Could you check a few things on this model? Use its own coordinates, in mm. Face numbers are marked on the shaded views. A direction names the side the tool comes from. Round coordinates to 2 decimals unless told otherwise and drop trailing zeros. Loops run counter-clockwise (first coordinate to the right, second up) from the corner with the lowest first, then second, coordinate; pieces in that order, holes last. Notation, with made-up numbers: M -37,8.25 L -28,8.25 A32 ccw -28,37.25 Z; hole C 70,32 d3. An arc over 180 degrees is marked long. One line per item, written item: value. Start each with the question number.
Q1. Imagine slicing it at B-B (x = 13). Please give me the cut outline in (y, z).
Q2. Thinking about a two-plate mould opening in Z: for the marked faces 1, 2 and 3, which applies, released by +Z, released by -Z, zero draft, split by the parting line, or undercut?
Q3. Please list where these lines run through material, in increasing order: line 1 along Z through (x, y) = (10.75, 40); line 2 along Z through (x, y) = (1, 4); line 3 along Y through (x, z) = (16, 1.65).
Q4. Imagine slicing it at A-A (z = 7). Please give me the cut outline in (x, y), then the cut area to 3 significant figures.
Q5. Imagine slicing it at D-D (z = 17.25). Please give me the cut outline in (x, y).
Q6. Imagine slicing it at C-C (y = 19). Please give me the cut outline in (x, z), then the cut area to 3 significant figures.
Q7. I'm going to push flat-ended pins straight in: pin 1 Ø2 at (y, z) = (40, 22) entering from -X; pin 2 Ø1.5 at (x, y) = (25.5, 25) entering from +Z; pin 3 Ø3 at (y, z) = (5, 21) entering from +X; pin 4 Ø1.5 at (x, z) = (24, 19) entering from -Y. Where does each tip first touch, or does it pass through?
Q8. Which directions (+Z, -Z, +X, -X, +Y, -Y) give clear straight access to the entire face, cutting with the end or side of a thin tool? Please do the marked faces 4, 5 and 6.
from build123d import *

# Parameters (mm, degrees)
SKETCH002_R     = 3.1
PAD001_DEPTH    = 20
PAD_DEPTH       = 30
SKETCH001_R     = 13
POCKET_DEPTH    = 27
SKETCH003_R     = 1.7
POCKET001_DEPTH = 3
SKETCH004_R     = 3.6
SKETCH004_R_2   = 1.7
POCKET002_DEPTH = 3


with BuildPart() as pad001:
    # Sketch002 → Pad001 (new body)
    with BuildSketch(Plane.YZ.offset(3)):
        with Locations((4, 22)):
            Circle(SKETCH002_R)
        with Locations((40, 22)):
            Circle(SKETCH002_R)
        with Locations((4, 8)):
            Circle(SKETCH002_R)
        with Locations((40, 8)):
            Circle(SKETCH002_R)
    extrude(amount=PAD001_DEPTH)


with BuildPart() as pocket002:
    # Sketch → Pad (new body)
    with BuildSketch(Plane.XY):
        with BuildLine():
            Line((0, 0), (0, 44))
            Line((0, 44), (3, 44))
            Line((3, 44), (21.975605, 35.758343))
            ThreePointArc((21.975609, 8.241648), (31, 21.999997), (21.975605, 35.758343))
            Line((21.975609, 8.241648), (3, 0))
            Line((3, 0), (0, 0))
        make_face()
    extrude(amount=PAD_DEPTH)

    # Sketch001 → Pocket (cut)
    with BuildSketch(Plane.XY.offset(30)):
        with Locations((16, 22)):
            Circle(SKETCH001_R)
    extrude(amount=-POCKET_DEPTH, mode=Mode.SUBTRACT)

    # Cut: cut Pad001
    add(pad001.part, mode=Mode.SUBTRACT)

    # Sketch003 → Pocket001 (cut)
    with BuildSketch(Plane.YZ.offset(3)):
        with Locations((4, 22)):
            Circle(SKETCH003_R)
        with Locations((40, 22)):
            Circle(SKETCH003_R)
        with Locations((4, 8)):
            Circle(SKETCH003_R)
        with Locations((40, 8)):
            Circle(SKETCH003_R)
    extrude(amount=-POCKET001_DEPTH, mode=Mode.SUBTRACT)

    # Sketch004 → Pocket002 (cut)
    with BuildSketch(Plane.XY.offset(3)):
        with Locations((16, 22)):
            Circle(SKETCH004_R)
        with Locations((16, 29.81356)):
            Circle(SKETCH004_R_2)
        with Locations((16, 14.18644)):
            Circle(SKETCH004_R_2)
    extrude(amount=-POCKET002_DEPTH, mode=Mode.SUBTRACT)


solid = pocket002.part
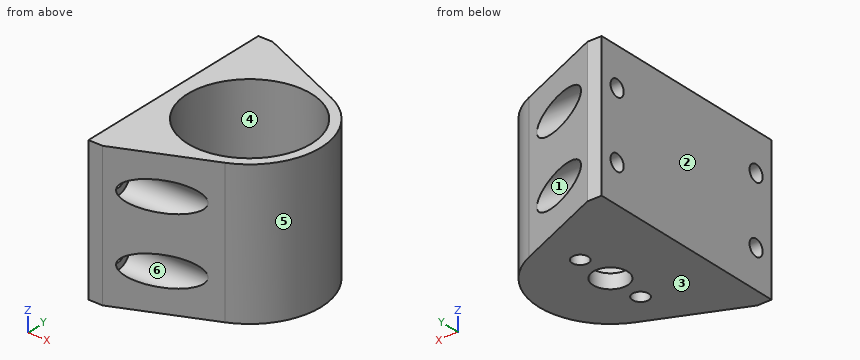
Report:
1. outline: M 4.34,0 L 20.01,0 L 20.01,3 L 9.35,3 L 9.35,30 L 4.34,30 L 4.34,25.08 A3.1 cw 4.34,18.92 L 4.34,11.08 A3.1 cw 4.34,4.92 Z; M 23.99,0 L 39.66,0 L 39.66,4.92 A3.1 cw 39.66,11.08 L 39.66,18.92 A3.1 cw 39.66,25.08 L 39.66,30 L 34.65,30 L 34.65,3 L 23.99,3 Z
2. face 1: undercut
2. face 2: zero draft
2. face 3: released by -Z
3. line 1: z = 0 to 4.9, 11.1 to 18.9, 25.1 to 30
3. line 2: z = 0 to 6.3, 9.7 to 20.3, 23.7 to 30
3. line 3: y = 5.65 to 12.49, 15.89 to 18.4, 25.6 to 28.11, 31.51 to 38.35
4. outline: M 0,0 L 3,0 L 5.45,1.07 L 3,1.07 L 3,2.63 L 0,2.63 Z; M 0,5.37 L 3,5.37 L 3,6.93 L 18.97,6.93 L 21.98,8.24 A15 ccw 21.98,35.76 L 18.97,37.07 L 3,37.07 L 3,38.63 L 0,38.63 Z; M 0,41.37 L 3,41.37 L 3,42.93 L 5.45,42.93 L 3,44 L 0,44 Z; hole C 16,22 d26
4. area: 334 mm²
5. outline: M 0,0 L 3,0 L 21.98,8.24 A15 ccw 21.98,35.76 L 3,44 L 0,44 Z; hole C 16,22 d26
6. outline: M 0,0 L 14.01,0 L 14.01,3 L 3.35,3 L 3.35,30 L 0,30 Z; M 17.99,0 L 30.7,0 L 30.7,30 L 28.65,30 L 28.65,3 L 17.99,3 Z
6. area: 226 mm²
7. pin 1: passes through
7. pin 2: stops at z = 3
7. pin 3: stops at x = 3
7. pin 4: stops at y = 8.87
8. face 4: +Z
8. face 5: +Z, -Z, +X
8. face 6: +X
